Could you check a few things on this model? Use its own coordinates, in mm. Face numbers are marked on the shaded views. A direction names the side the tool comes from. Round coordinates to 2 decimals unless told otherwise and drop trailing zeros. Loops run counter-clockwise (first coordinate to the right, second up) from the corner with the lowest first, then second, coordinate; pieces in that order, holes last. Notation, with made-up numbers: (-23, -6) -> (-9, -6) arc R24 cw to (-9, 26) -> close; hole circle Ø7 at (72, 12). An arc over 180 degrees is marked (long way). One line per item, written item: value.
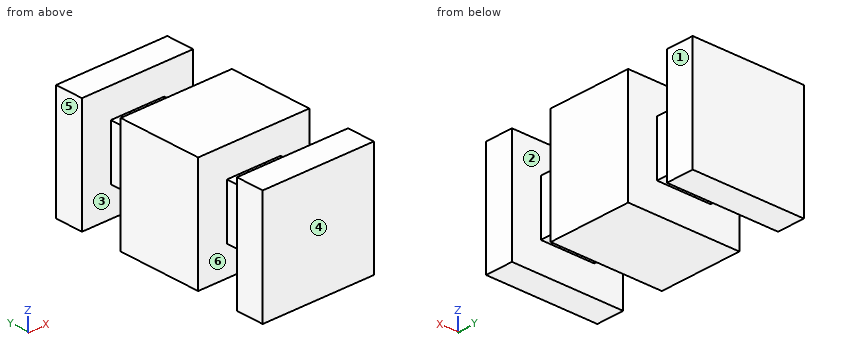
```python
from build123d import *

# Parameters (mm, degrees)
F0_W      = 8
F0_H      = 6
F1_DEPTH  = 8
F2_W      = 3.85
F2_H      = 3.85
F3_DEPTH  = 3
F4_W      = 8
F4_H      = 8
F4_W_2    = 3.85
F4_H_2    = 3.85
F5_DEPTH  = 2
F7_W      = 3.85
F7_H      = 3.85
F8_DEPTH  = 3
F9_W      = 8
F9_H      = 8
F9_W_2    = 3.85
F9_H_2    = 3.85
F10_DEPTH = 2.35
F11_DEPTH = 0.35


with BuildPart() as f1:
    # F0 (on Top) → F1 (new body)
    with BuildSketch(Plane.XY):
        Rectangle(F0_W, F0_H)
    extrude(amount=F1_DEPTH)

    # F2 (on face) → F3 (join)
    with BuildSketch(Plane.XZ.offset(3)):
        with Locations((0, 4)):
            Rectangle(F2_W, F2_H)
    extrude(amount=F3_DEPTH)

    # F4 (on face) → F5 (join)
    with BuildSketch(Plane.XZ.offset(6)):
        with Locations((0, 4)):
            Rectangle(F4_W, F4_H)
        with Locations((0, 4)):
            Rectangle(F4_W_2, F4_H_2, mode=Mode.SUBTRACT)
        with Locations((0, 4)):
            Rectangle(F4_W_2, F4_H_2)
    extrude(amount=F5_DEPTH)

    # F7 (on face) → F8 (join)
    with BuildSketch(Plane(origin=(0, 3, 0), x_dir=(-1, 0, 0), z_dir=(0, 1, 0))):
        with Locations((0, 4)):
            Rectangle(F7_W, F7_H)
    extrude(amount=F8_DEPTH)

    # F9 (on face) → F10 (join)
    with BuildSketch(Plane(origin=(0, 6, 0), x_dir=(-1, 0, 0), z_dir=(0, 1, 0))):
        with Locations((0, 4)):
            Rectangle(F9_W, F9_H)
        with Locations((0, 4)):
            Rectangle(F9_W_2, F9_H_2, mode=Mode.SUBTRACT)
        with Locations((0, 4)):
            Rectangle(F9_W_2, F9_H_2)
    extrude(amount=F10_DEPTH)

    # F11 (cut): a face of the model
    f11_faces = [f1.faces().sort_by_distance(p)[0] for p in [
        (0, 8.35, 4),
    ]]
    extrude(f11_faces, amount=-F11_DEPTH, mode=Mode.SUBTRACT)


solid = f1.part
```
(1) Imagine slicing it at B-B on z = 6.5. Write out the boundary of the cut face in (x, y).
Results below:
outline: (-4, -8) -> (4, -8) -> (4, -6) -> (-4, -6) -> close; (-4, -3) -> (4, -3) -> (4, 3) -> (-4, 3) -> close; (-4, 6) -> (4, 6) -> (4, 8) -> (-4, 8) -> close
(2) Please list where these lines run through material, in increasing order: L1, parallel to Y at x = -3.5, z = 4.25; L2, parallel to X at y = -4.25, z = 3 (3 decimals); L3, parallel to Z at x = -1, y = -4.25 (3 decimals).
Results below:
L1: y = -8 to -6, -3 to 3, 6 to 8
L2: x = -1.925 to 1.925
L3: z = 2.075 to 5.925
(3) Imagine slicing it at D-D on x = -0.5. Write out the boundary of the cut face in (y, z) (3 decimals), then the cut area to 3 significant figures.
Results below:
outline: (-8, 0) -> (-6, 0) -> (-6, 2.075) -> (-3, 2.075) -> (-3, 0) -> (3, 0) -> (3, 2.075) -> (6, 2.075) -> (6, 0) -> (8, 0) -> (8, 8) -> (6, 8) -> (6, 5.925) -> (3, 5.925) -> (3, 8) -> (-3, 8) -> (-3, 5.925) -> (-6, 5.925) -> (-6, 8) -> (-8, 8) -> close
area: 103 mm²
(4) For pin 1 Ø1.5 at (x, y) = (0.5, -4) entering from -Z (3 decimals); pin 2 Ø1.5 at (x, y) = (1, 4) entering from +Z (3 decimals); pin 3 Ø1.5 at (y, z) = (-4.5, 4) entering from -X (3 decimals), each with a flat end and sliding along its axis, tell me the tip position at first contact or that it passes through.
Results below:
pin 1: stops at z = 2.075
pin 2: stops at z = 5.925
pin 3: stops at x = -1.925
(5) On a 3-axis mill with a long thin cutter (end or side, diameter ignored), from which of +Z, -Z, +X, -X, +Y, -Y can I reach the whole of each face in a straight line? I mean the marked faces 1 and 2. Say none if no direction works.
Results below:
face 1: +Z, -Z, +X, +Y, -Y
face 2: none
(6) Imagine slicing it at C-C on z = 4. Write out the boundary of the cut face in (x, y) (3 decimals).
Results below:
outline: (-4, -8) -> (4, -8) -> (4, -6) -> (1.925, -6) -> (1.925, -3) -> (4, -3) -> (4, 3) -> (1.925, 3) -> (1.925, 6) -> (4, 6) -> (4, 8) -> (-4, 8) -> (-4, 6) -> (-1.925, 6) -> (-1.925, 3) -> (-4, 3) -> (-4, -3) -> (-1.925, -3) -> (-1.925, -6) -> (-4, -6) -> close
(7) We'd pull the mould along Y, two halves only. Please class the marked faces 3, 4, 5 and 6: +Y half, -Y half, draft (parallel to the pull), parting line (faces both ways), or undercut.
Results below:
face 3: undercut
face 4: -Y half
face 5: draft
face 6: undercut
(8) Imagine slicing it at A-A on x = 2.25. Write out the boundary of the cut face in (y, z).
Results below:
outline: (-8, 0) -> (-6, 0) -> (-6, 8) -> (-8, 8) -> close; (-3, 0) -> (3, 0) -> (3, 8) -> (-3, 8) -> close; (6, 0) -> (8, 0) -> (8, 8) -> (6, 8) -> close
